Model file for the job. Use its own axes, mm. Give positions to 0.01 mm unless a question says otherwise; leave off trailing zeros. Write each loop counter-clockwise with the first axis right and the second up, starting at its lowest first coordinate (ties: lowest second). Pieces come first, ordered by that corner, then holes.
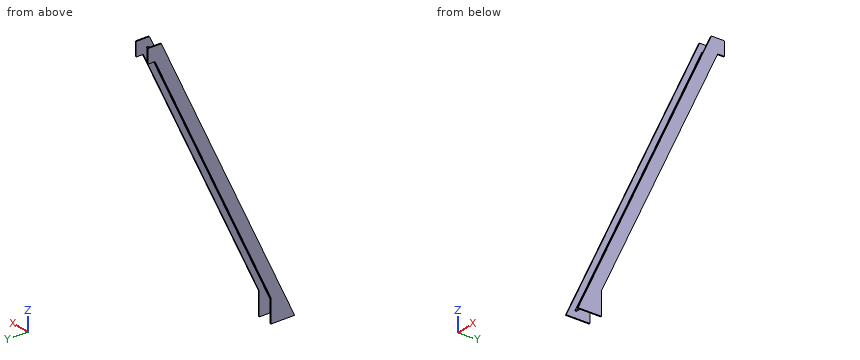
```python
from build123d import *

# Parameters (mm, degrees)
F2_DEPTH      = 1
F5_DEPTH      = 6
F5_DEPTH_BACK = 6


with BuildPart() as f2:
    # F1 (on offset) → F2 (new body)
    with BuildSketch(Plane.YZ.offset(-7)):
        Polygon((115.177992, 247), (0, 0), (20.359932, 0), (20.359932, 20), (120.616079, 235), (126.616079, 235), (126.616079, 247), align=None)
    extrude(amount=F2_DEPTH)



with BuildPart() as f3_1:
    # F3: instance of F2
    add(f2.part.mirror(Plane.YZ))


with BuildPart() as f2_1:
    add(f2.part)

    add(f3_1.part)  # F5 merges F3_1
    # F4 (on Right) → F5 (join, two sides)
    with BuildSketch(Plane.YZ) as f5_sk:
        Polygon((117.834365, 239.682502), (116.928057, 240.10512), (7.607535, 5.666504), (8.513843, 5.243886), align=None)
    extrude(amount=F5_DEPTH)
    extrude(f5_sk.sketch, amount=-F5_DEPTH_BACK)


solid = f2_1.part
```
1. Slice it at C-C, the plane y = 104.5. Write the cut outline in (x, z).
Calculated:
outline: (-7, 200.44) - (-6, 200.44) - (-6, 211.09) - (6, 211.09) - (6, 200.44) - (7, 200.44) - (7, 224.1) - (6, 224.1) - (6, 213.45) - (-6, 213.45) - (-6, 224.1) - (-7, 224.1) - close
2. Pin check, flat tips, straight feed: P1, Ø3, axis at x = -1.5, z = 167.5, coming from the -Y side; P2, Ø1.5, axis at x = -3.5, y = 82.5, coming from the -Z side; P3, Ø0.8, axis at x = -6.5, y = 125, coming from the -Z side. Stop position of each tip, or through.
Calculated:
P1: stops at y = 82.37
P2: stops at z = 162.3
P3: stops at z = 235
3. Slice it at B-B, the plane x = 3. Write the cut outline in (y, z).
Calculated:
outline: (7.61, 5.67) - (8.51, 5.24) - (117.83, 239.68) - (116.93, 240.11) - close
4. Probe probe 1 along X at (y, z) = (97.5, 188); probe 2 along Y at (x, z) = (4.25, 157); probe 3 along Y at (x, z) = (2.5, 35). List the from-to ranges inside material, lowest first.
Calculated:
probe 1: x = -7 to -6, 6 to 7
probe 2: y = 78.18 to 79.28
probe 3: y = 21.29 to 22.39
5. Slice it at A-A, the plane z = 184.5. Write the cut outline in (x, y).
Calculated:
outline: (-7, 86.03) - (-6, 86.03) - (-6, 91) - (6, 91) - (6, 86.03) - (7, 86.03) - (7, 97.07) - (6, 97.07) - (6, 92.1) - (-6, 92.1) - (-6, 97.07) - (-7, 97.07) - close
